```python
from build123d import *

# Parameters (mm, degrees)
BOSS_EXTRUDE1_DEPTH  = 1.5
M3_CLEARANCE_HOLE1_D = 3.4
SKETCH4_R            = 1.55
CUT_EXTRUDE1_DEPTH   = 2.5


with BuildPart() as part:
    # Sketch1 → Boss-Extrude1 (new body)
    with BuildSketch(Plane(origin=(0, 0, 0), x_dir=(1, 0, 0), z_dir=(0, 1, 0))):
        with BuildLine():
            Line((0, 4), (45, 4))
            ThreePointArc((45, 4), (49, 0), (45, -4))
            Line((45, -4), (0, -4))
            ThreePointArc((0, -4), (-4, 0), (0, 4))
        make_face()
    extrude(amount=BOSS_EXTRUDE1_DEPTH)

    # M3 Clearance Hole1 (through all)
    with Locations(Plane(origin=(0, 1.5, 0), x_dir=(1, 0, 0), z_dir=(0, 1, 0))):
        with Locations((0, 0)):
            Hole(M3_CLEARANCE_HOLE1_D / 2)

    # Sketch4 → Cut-Extrude1 (cut, through all)
    with BuildSketch(Plane(origin=(0, 1.5, 0), x_dir=(1, 0, 0), z_dir=(0, 1, 0))):
        with Locations((45, 0)):
            Circle(SKETCH4_R)
    extrude(amount=-CUT_EXTRUDE1_DEPTH, mode=Mode.SUBTRACT)


solid = part.part
```
Model file for the job. Use its own axes, mm. Coordinates: 2 decimals unless noted, no trailing zeros. Loops run counter-clockwise (first coordinate to the right, second up) from the corner with the lowest first, then second, coordinate; pieces in that order, holes last. Notation, with made-up numbers: (40, -16.5) - (85, -16.5) arc R19 cw to (85, -8.5) - close; hole circle Ø1 at (47.25, -15.75). An arc over 180 degrees is marked (long way). Answer as a JSON object with one key per item and string values. Group by question number.
(1) Cut at C-C (x = 44.5). Give the cut face in (y, z).
(2) Cut at D-D (z = -2.5). Give the cut face in (x, y).
(3) Cut at B-B (y = 1.25). Give the cut face in (x, z), then the cut area to 3 significant figures.
(4) Probe line 1 along Z through (x, y) = (45, 1.2); line 2 along Z through (x, y) = (0, 0.5); line 3 along X through (y, z) = (1.25, -0.25). List the from-to ranges inside material, lowest first.
(5) Two-plate mould, pull along Z, no slides. Class faces 1 (the face through (46.478, 0.76, -0.466)), 2 (the face through (-4, 1, 0)), 3 (the face through (22, 1, -4)), 4 (the face through (23, 1, 4)): released by +Z, released by -Z, zero draft, split by the parting line, or undercut.
(6) Cut at A-A (z = 0). Give the cut face in (x, y).
Geometry says:
{
 "1": {"outline": "(0, -4) - (1.5, -4) - (1.5, -1.47) - (0, -1.47) - close; (0, 1.47) - (1.5, 1.47) - (1.5, 4) - (0, 4) - close"},
 "2": {"outline": "(-3.12, 0) - (48.12, 0) - (48.12, 1.5) - (-3.12, 1.5) - close"},
 "3": {"outline": "(0, -4) - (45, -4) arc R4 ccw to (45, 4) - (0, 4) arc R4 ccw to start; hole circle Ø3.4 at (0, 0); hole circle Ø3.1 at (45, 0)", "area": "394 mm^2"},
 "4": {"line 1": "z = -4 to -1.55, 1.55 to 4", "line 2": "z = -4 to -1.7, 1.7 to 4", "line 3": "x = -3.99 to -1.68, 1.68 to 43.47, 46.53 to 48.99"},
 "5": {"face 1": "undercut", "face 2": "split by the parting line", "face 3": "released by -Z", "face 4": "released by +Z"},
 "6": {"outline": "(-4, 0) - (-1.7, 0) - (-1.7, 1.5) - (-4, 1.5) - close; (1.7, 0) - (43.45, 0) - (43.45, 1.5) - (1.7, 1.5) - close; (46.55, 0) - (49, 0) - (49, 1.5) - (46.55, 1.5) - close"}
}
